from build123d import *

# Parameters (mm, degrees)
ESBO_O1_W                = 12
ESBO_O1_H                = 17
ESBO_O1_R                = 1.65
RESSALTO_EXTRUS_O1_DEPTH = 1.5
ESBO_O2_R                = 2.5
ESBO_O2_W                = 5
ESBO_O2_H                = 5.148031572
RESSALTO_EXTRUS_O2_DEPTH = 1.5


with BuildPart() as part:
    # Esboço1 → Ressalto-extrusão1 (new body)
    with BuildSketch(Plane.XY):
        Rectangle(ESBO_O1_W, ESBO_O1_H)
        with Locations((3.652764924, -5.682274929)):
            Circle(ESBO_O1_R, mode=Mode.SUBTRACT)
    extrude(amount=RESSALTO_EXTRUS_O1_DEPTH)

    # Esboço2 → Ressalto-extrusão2 (add)
    with BuildSketch(Plane.XY.offset(1.5)):
        with Locations((-3.353706204, 3.998787781)):
            Circle(ESBO_O2_R)
        with Locations((2.646293796, 3.998787781)):
            Rectangle(ESBO_O2_W, ESBO_O2_H)
    extrude(amount=RESSALTO_EXTRUS_O2_DEPTH)


solid = part.part
Geometry check sheet. Reference: the model listing, model coordinates, mm. A direction names the side the tool comes from. Round coordinates to 2 decimals unless told otherwise and drop trailing zeros. Order: outer loops, then holes, each group sorted by start corner. A loop starts at its lowest first (then second) coordinate and runs counter-clockwise, first axis right, second up. Notation, with made-up numbers: (8.25, 1) -> (19.25, 1) arc R32 cw to (19.25, 28) -> close; hole circle Ø1 at (73.25, 65). An arc over 180 degrees is marked (long way). Use one line per item in the form item = value.
1. Cross-section at D-D, the plane x = 0.75. Enter the section's corners in (y, z), plus the area to 3 significant figures.
Working result:
outline = (-8.5, 0) -> (8.5, 0) -> (8.5, 1.5) -> (6.57, 1.5) -> (6.57, 3) -> (1.42, 3) -> (1.42, 1.5) -> (-8.5, 1.5) -> close
area = 33.2 mm^2
2. Cross-section at C-C, the plane z = 1.95. Enter the section's corners in (x, y).
Working result:
outline = circle Ø5 at (-3.35, 4); (0.15, 1.42) -> (5.15, 1.42) -> (5.15, 6.57) -> (0.15, 6.57) -> close
3. Set-up check for faces 4 (the face through (-5.85, 4.11, 2.24)), 5 (the face through (3, 6.573, 2)), 6 (the face through (3, 1.425, 2)), 7 (the face through (5.146, 4, 2)): record each of +Z, -Z, +X, -X, +Y, -Y from which the full face is reachable in a straight line by a thin tool's end or side.
Working result:
face_4 = +Z
face_5 = +Z, +X, -X, +Y
face_6 = +Z, +X, -X, -Y
face_7 = +Z, +X, +Y, -Y
4. Cross-section at A-A, the plane x = 4.75. Enter the section's corners in (y, z), plus the area to 3 significant figures.
Working result:
outline = (-8.5, 0) -> (-6.91, 0) -> (-6.91, 1.5) -> (-8.5, 1.5) -> close; (-4.45, 0) -> (8.5, 0) -> (8.5, 1.5) -> (6.57, 1.5) -> (6.57, 3) -> (1.42, 3) -> (1.42, 1.5) -> (-4.45, 1.5) -> close
area = 29.5 mm^2
5. Mould release check, pull along X, two halves, no side actions. Record for faces 1 (the face through (-6, 0, 1)), 2 (the face through (0.146, 4, 2)), 3 (the face through (0, 8.5, 1)): pulls with the +X half, pulls with the -X half, needs draft (parallel to the pull), parting line crosses it, or undercut.
Working result:
face_1 = pulls with the -X half
face_2 = undercut
face_3 = needs draft
6. Scan lines: line 1 along Z through (x, y) = (-4.5, -1.5); line 2 along X through (y, z) = (1.75, 1.6); line 3 along X through (y, z) = (5, 1.55). Record each from-to range of solid material in increasing order. Write a range as from..to.
Working result:
line_1 = 0..1.5
line_2 = -4.45..-2.26, 0.15..5.15
line_3 = -5.64..-1.06, 0.15..5.15
7. Go/stop test with flat-tipped pins: pin 1 (0.8 mm diameter, centred on x = 3, z = 2, fed in from -Y); pin 2 (1.2 mm diameter, centred on x = 2, z = 2.5, fed in from +Y); pin 3 (0.8 mm diameter, centred on y = 4, z = 2.5, fed in from -X). Record where each tip stops, or that it passes through.
Working result:
pin_1 = 1.42
pin_2 = 6.57
pin_3 = -5.85
8. Cross-section at B-B, the plane y = -6. Enter the section's corners in (x, z).
Working result:
outline = (-6, 0) -> (2.03, 0) -> (2.03, 1.5) -> (-6, 1.5) -> close; (5.27, 0) -> (6, 0) -> (6, 1.5) -> (5.27, 1.5) -> close
